```python
from build123d import *

# Parameters (mm, degrees)
SKIZZE1_W                            = 6
SKIZZE1_H                            = 6
AUFSATZ_LINEAR_AUSTRAGEN1_DEPTH      = 1.5
SKIZZE2_W                            = 5
SKIZZE2_H                            = 5
AUFSATZ_LINEAR_AUSTRAGEN2_DEPTH      = 3
SKIZZE3_W                            = 4
SKIZZE3_H                            = 4
SCHNITT_LINEAR_AUSTRAGEN1_DEPTH      = 3.5
VERRUNDUNG1_R                        = 1
VERRUNDUNG2_R                        = 1.5
VERRUNDUNG3_R                        = 1.5
FASE1_SIZE                           = 0.1
F_0_2_0_2_DURCHMESSER_BOHRUNG5_D     = 0.2
F_0_2_0_2_DURCHMESSER_BOHRUNG5_DEPTH = 0.01
F_0_2_0_2_DURCHMESSER_BOHRUNG5_TIP   = 0.1
SKIZZE7_R                            = 2.25
SCHNITT_LINEAR_AUSTRAGEN2_DEPTH      = 0.5


with BuildPart() as part:
    # Skizze1 → Aufsatz-Linear austragen1 (new body)
    with BuildSketch(Plane.XY):
        Rectangle(SKIZZE1_W, SKIZZE1_H)
    extrude(amount=-AUFSATZ_LINEAR_AUSTRAGEN1_DEPTH)

    # Skizze2 → Aufsatz-Linear austragen2 (add)
    with BuildSketch(Plane(origin=(0, 0, 0), x_dir=(-1, 0, 0), z_dir=(0, 0, -1))):
        Rectangle(SKIZZE2_W, SKIZZE2_H)
    extrude(amount=-AUFSATZ_LINEAR_AUSTRAGEN2_DEPTH)

    # Skizze3 → Schnitt-Linear austragen1 (cut)
    with BuildSketch(Plane.XY.offset(3)):
        Rectangle(SKIZZE3_W, SKIZZE3_H)
    extrude(amount=-SCHNITT_LINEAR_AUSTRAGEN1_DEPTH, mode=Mode.SUBTRACT)

    # Verrundung1
    verrundung1_edges = [part.edges().sort_by_distance(p)[0] for p in [
        (2, 2, 1.25),
        (2, -2, 1.25),
        (-2, -2, 1.25),
        (-2, 2, 1.25),
    ]]
    fillet(verrundung1_edges, radius=VERRUNDUNG1_R)

    # Verrundung2
    verrundung2_edges = [part.edges().sort_by_distance(p)[0] for p in [
        (-2.5, 2.5, 1.5),
        (-2.5, -2.5, 1.5),
        (2.5, -2.5, 1.5),
        (2.5, 2.5, 1.5),
    ]]
    fillet(verrundung2_edges, radius=VERRUNDUNG2_R)

    # Verrundung3
    verrundung3_edges = [part.edges().sort_by_distance(p)[0] for p in [
        (3, -3, -0.75),
        (-3, -3, -0.75),
        (-3, 3, -0.75),
        (3, 3, -0.75),
    ]]
    fillet(verrundung3_edges, radius=VERRUNDUNG3_R)

    # Fase1
    fase1_edges = [part.edges().sort_by_distance(p)[0] for p in [
        (0, -2, 3),
        (-2, 0, 3),
        (2, 0, 3),
        (0, 2, 3),
        (-1.707106781, -1.707106781, 3),
        (1.707106781, -1.707106781, 3),
        (1.707106781, 1.707106781, 3),
        (-1.707106781, 1.707106781, 3),
        (0, -2.5, 0),
        (0, -2.5, 3),
        (-2.5, 0, 0),
        (-2.5, 0, 3),
        (2.5, 0, 3),
        (0, 2.5, 3),
        (-2.060660172, 2.060660172, 3),
        (2.060660172, 2.060660172, 3),
        (2.060660172, -2.060660172, 3),
        (-2.060660172, -2.060660172, 3),
        (2.5, 0, 0),
        (0, 2.5, 0),
        (-2.060660172, -2.060660172, 0),
        (2.060660172, -2.060660172, 0),
        (2.060660172, 2.060660172, 0),
        (-2.060660172, 2.060660172, 0),
        (-3, 0, 0),
        (3, 0, 0),
        (0, 3, 0),
        (0, -3, 0),
        (-2.560660172, 2.560660172, 0),
        (2.560660172, 2.560660172, 0),
        (2.560660172, -2.560660172, 0),
        (-2.560660172, -2.560660172, 0),
    ]]
    chamfer(fase1_edges, length=FASE1_SIZE)

    # Ø0.2 (0.2) Durchmesser Bohrung5
    with Locations(Plane(origin=(2.060660172, 2.060660172, 0), x_dir=(0.707106781, -0.707106781, 0), z_dir=(0.707106781, 0.707106781, 0))):
        with Locations((0, -1.6)):
            Hole(F_0_2_0_2_DURCHMESSER_BOHRUNG5_D / 2, depth=F_0_2_0_2_DURCHMESSER_BOHRUNG5_DEPTH)
            with Locations((0, 0, -(F_0_2_0_2_DURCHMESSER_BOHRUNG5_DEPTH + F_0_2_0_2_DURCHMESSER_BOHRUNG5_TIP / 2))):  # 90° drill point
                Cone(0, F_0_2_0_2_DURCHMESSER_BOHRUNG5_D / 2, F_0_2_0_2_DURCHMESSER_BOHRUNG5_TIP, mode=Mode.SUBTRACT)

    # Skizze7 → Schnitt-Linear austragen2 (cut)
    with BuildSketch(Plane.XY):
        with Locations((-4.85, 0)):
            Circle(SKIZZE7_R)
        with Locations((4.85, 0)):
            Circle(SKIZZE7_R)
    extrude(amount=-SCHNITT_LINEAR_AUSTRAGEN2_DEPTH, mode=Mode.SUBTRACT)


solid = part.part
```
Work out the finished part from the listing and answer in its coordinate system (mm). A direction names the side the tool comes from. Round coordinates to 2 decimals unless told otherwise and drop trailing zeros. Write each loop counter-clockwise with the first axis right and the second up, starting at its lowest first coordinate (ties: lowest second). Pieces come first, ordered by that corner, then holes.
1) Which of the six approach directions +Z, -Z, +X, -X, +Y, -Y give full straight-line access (tool end or side, diameter ignored) to faces 1 (the face through (3, 0, -1)), 2 (the face through (2.07, -2.05, 1.52)), 3 (the face through (-2.05, 2.07, 1.52)), 4 (the face through (-1.715, 1.699, 1.176)), 5 (the face through (0, 2.5, 1))?
2) Determine the mould class of faces 6 (the face through (2, 0, 1)), 7 (the face through (-2.57, 2.55, -0.81)), 8 (the face through (0, -2.5, 1)) for opening direction X: pulls with the +X half, pulls with the -X half, needs draft (parallel to the pull), parting line crosses it, or undercut.
3) A cutting plane is placed at C-C on z = -0.9. Determine the outline of the cut face in (x, y).
4) A cutting plane is placed at B-B on x = 0. Determine the outline of the cut face in (y, z).
5) A cutting plane is placed at A-A on z = -0.2. Determine the outline of the cut face in (x, y).
6) Flat-ended cylindrical pins translate along their axes: P1, Ø1.2, axis at x = 0, y = -0.5, coming from the +Z side; P2, Ø1, axis at x = 0.5, z = 2, coming from the +Y side; P3, Ø0.6, axis at y = 0, z = 1, coming from the -X side. Find the tip coordinate at first contact, or state that the pin passes through.
7) A cutting plane is placed at D-D on y = 0.85. Determine the outline of the cut face in (x, z), and give its area (3 significant figures).
8) Consider probe 1 along X at (y, z) = (-0.4, 2.25); probe 2 along Z at (x, y) = (0, 0.3). Determine where each line is inside the solid, lowest interval first.
Entries:
1. face 1: +Z, -Z, +X, +Y, -Y
1. face 2: +Z, +X, -Y
1. face 3: +Z, -X, +Y
1. face 4: +Z
1. face 5: +Z, +X, -X, +Y
2. face 6: undercut
2. face 7: pulls with the -X half
2. face 8: needs draft
3. outline: (-3, -1.5) arc R1.5 ccw to (-1.5, -3) - (1.5, -3) arc R1.5 ccw to (3, -1.5) - (3, 1.5) arc R1.5 ccw to (1.5, 3) - (-1.5, 3) arc R1.5 ccw to (-3, 1.5) - close
4. outline: (-3, -1.5) - (3, -1.5) - (3, -0.1) - (2.9, 0) - (2.6, 0) - (2.5, 0.1) - (2.5, 2.9) - (2.4, 3) - (2.1, 3) - (2, 2.9) - (2, -0.5) - (-2, -0.5) - (-2, 2.9) - (-2.1, 3) - (-2.4, 3) - (-2.5, 2.9) - (-2.5, 0.1) - (-2.6, 0) - (-2.9, 0) - (-3, -0.1) - close
5. outline: (-3, -1.5) arc R1.5 ccw to (-1.5, -3) - (1.5, -3) arc R1.5 ccw to (3, -1.5) - (3, -1.28) arc R2.25 cw to (3, 1.28) - (3, 1.5) arc R1.5 ccw to (1.5, 3) - (-1.5, 3) arc R1.5 ccw to (-3, 1.5) - (-3, 1.28) arc R2.25 cw to (-3, -1.28) - close; hole (-2, -1) arc R1 ccw to (-1, -2) - (1, -2) arc R1 ccw to (2, -1) - (2, 1) arc R1 ccw to (1, 2) - (-1, 2) arc R1 ccw to (-2, 1) - close
6. P1: stops at z = -0.5
6. P2: stops at y = 2.5
6. P3: stops at x = -2.5
7. outline: (-3, -1.5) - (3, -1.5) - (3, -0.5) - (2.77, -0.5) - (2.77, 0) - (2.6, 0) - (2.5, 0.1) - (2.5, 2.9) - (2.4, 3) - (2.1, 3) - (2, 2.9) - (2, -0.5) - (-2, -0.5) - (-2, 2.9) - (-2.1, 3) - (-2.4, 3) - (-2.5, 2.9) - (-2.5, 0.1) - (-2.6, 0) - (-2.77, 0) - (-2.77, -0.5) - (-3, -0.5) - close
7. area: 9.76 mm2
8. probe 1: x = -2.5 to -2, 2 to 2.5
8. probe 2: z = -1.5 to -0.5
